Verification items for the finished model (mm, model axes). Coordinates: 2 decimals unless noted, no trailing zeros. Write each loop counter-clockwise with the first axis right and the second up, starting at its lowest first coordinate (ties: lowest second). Pieces come first, ordered by that corner, then holes. Notation, with made-up numbers: M 59.25,78.25 L 83.25,78.25 A25 cw 83.25,112.25 Z; hole C -2.5,59 d4. An arc over 180 degrees is marked long. One line per item, written item: value.
```python
from build123d import *

# Parameters (mm, degrees)
SKETCH1_W           = 313
SKETCH1_H           = 342
BOSS_EXTRUDE1_DEPTH = 6.35
SKETCH3_W           = 22
SKETCH3_H           = 155.14040353
SKETCH3_R           = 2.5
BOSS_EXTRUDE2_DEPTH = 6.35
SKETCH2_R           = 2.5
CUT_EXTRUDE1_DEPTH  = 7.35
SKETCH4_R           = 3.5
CUT_EXTRUDE2_DEPTH  = 7.35
SKETCH5_R           = 1.5
SKETCH5_R_2         = 1.05
CUT_EXTRUDE3_DEPTH  = 7.35


with BuildPart() as part:
    # Sketch1 → Boss-Extrude1 (new body)
    with BuildSketch(Plane(origin=(0, 0, 0), x_dir=(1, 0, 0), z_dir=(0, 1, 0))):
        Rectangle(SKETCH1_W, SKETCH1_H)
    extrude(amount=-BOSS_EXTRUDE1_DEPTH)

    # Sketch3 → Boss-Extrude2 (add)
    with BuildSketch(Plane(origin=(0, 0, 0), x_dir=(1, 0, 0), z_dir=(0, 1, 0))):
        with Locations((167.5, 9)):
            Rectangle(SKETCH3_W, SKETCH3_H)
        with Locations((166.5, 9)):
            Circle(SKETCH3_R, mode=Mode.SUBTRACT)
        with Locations((166.5, -41.8)):
            Circle(SKETCH3_R, mode=Mode.SUBTRACT)
        with Locations((166.5, 59.8)):
            Circle(SKETCH3_R, mode=Mode.SUBTRACT)
    extrude(amount=-BOSS_EXTRUDE2_DEPTH)

    # Sketch2 → Cut-Extrude1 (cut, through all)
    with BuildSketch(Plane(origin=(0, 0, 0), x_dir=(1, 0, 0), z_dir=(0, 1, 0))):
        with Locations((0, -123)):
            Circle(SKETCH2_R)
        with Locations((-70, -123)):
            Circle(SKETCH2_R)
        with Locations((70, -123)):
            Circle(SKETCH2_R)
        with Locations((-70, 141)):
            Circle(SKETCH2_R)
        with Locations((0, 141)):
            Circle(SKETCH2_R)
        with Locations((70, 141)):
            Circle(SKETCH2_R)
    extrude(amount=-CUT_EXTRUDE1_DEPTH, mode=Mode.SUBTRACT)

    # Sketch4 → Cut-Extrude2 (cut, through all)
    with BuildSketch(Plane(origin=(0, 0, 0), x_dir=(1, 0, 0), z_dir=(0, 1, 0))):
        with Locations((133.64, -142.84)):
            Circle(SKETCH4_R)
        with Locations((108.24, -142.84)):
            Circle(SKETCH4_R)
    cut_extrude2 = extrude(amount=-CUT_EXTRUDE2_DEPTH, mode=Mode.SUBTRACT)

    # Mirror1: Cut-Extrude2 across plane
    add(cut_extrude2.mirror(Plane(origin=(0, 0, -9), x_dir=(1, 0, 0), z_dir=(0, 0, -1))), mode=Mode.SUBTRACT)

    # Sketch5 → Cut-Extrude3 (cut, through all)
    with BuildSketch(Plane(origin=(0, 0, 0), x_dir=(1, 0, 0), z_dir=(0, 1, 0))):
        with Locations((79.770037453, -148.470411985)):
            Circle(SKETCH5_R)
        with Locations((-6.229962547, -148.470411985)):
            Circle(SKETCH5_R)
        with Locations((-6.229962547, -12.470411985)):
            Circle(SKETCH5_R)
        with Locations((79.770037453, -12.470411985)):
            Circle(SKETCH5_R)
        with Locations((-46.113857678, -7.113857678)):
            Circle(SKETCH5_R_2)
        with Locations((-46.113857678, -152.113857678)):
            Circle(SKETCH5_R_2)
        with Locations((-141.113857678, -7.113857678)):
            Circle(SKETCH5_R_2)
        with Locations((-141.113857678, -152.113857678)):
            Circle(SKETCH5_R_2)
    extrude(amount=-CUT_EXTRUDE3_DEPTH, mode=Mode.SUBTRACT)


solid = part.part
```
Item 1: Cross-section at B-B, the plane z = 86. Enter the section's corners in (x, y).
The answers:
outline: M -156.5,-6.35 L 156.5,-6.35 L 156.5,0 L -156.5,0 Z
Item 2: Scan lines: line 1 (Z direction, x = 108, y = -1); line 2 (Z direction, x = 70, y = -4); line 3 (X direction, y = -2.25, z = -141). Record each from-to range of solid material in increasing order.
The answers:
line 1: z = -171 to -164.33, -157.35 to 139.35, 146.33 to 171
line 2: z = -171 to -143.5, -138.5 to 120.5, 125.5 to 171
line 3: x = -156.5 to -72.5, -67.5 to -2.5, 2.5 to 67.5, 72.5 to 156.5
Item 3: Cross-section at A-A, the plane y = -3.5. Give the number of separate pieces and of enclosed holes in the cut face, and give its area (3 significant figures).
The answers:
separate pieces: 1
enclosed holes: 21
area: 110,000 mm²
Item 4: Go/stop test with flat-tipped pins: P1, Ø2.5, axis at x = -141.11, z = 7.11, coming from the -Y side; P2, Ø1.7, axis at x = -46.11, z = 7.11, coming from the +Y side. Record where each tip stops, or that it passes through.
The answers:
P1: stops at y = -6.35
P2: passes through
